```python
from build123d import *

# Parameters (mm, degrees)
FILLET1_R = 3


with BuildPart() as part:
    # Sketch1 → Revolve1 (revolve)
    with BuildSketch(Plane(origin=(0, 0, 0), x_dir=(0, 0, -1), z_dir=(1, 0, 0))):
        Polygon((-26, 0), (-15, 0), (-15, 2), (0, 2), (0, 12.5), (-4, 12.5), (-26, 9.408101637), align=None)
    revolve(axis=Axis((0, 0, 0), (0, 0, 1)))

    # Fillet1
    fillet1_edges = [part.edges().sort_by_distance(p)[0] for p in [
        (0, -9.408101637, 26),
        (0, -12.5, 4),
    ]]
    fillet(fillet1_edges, radius=FILLET1_R)


solid = part.part
```
Here's how the part is built. I have some questions about the finished solid (model axes, mm). Coordinates: 2 decimals unless noted, no trailing zeros. Order: outer loops, then holes, each group sorted by start corner. A loop starts at its lowest first (then second) coordinate and runs counter-clockwise, first axis right, second up.
1) Imagine slicing it at B-B on z = 23. List the corners of the cut face in (x, y) for me.
2) Imagine slicing it at A-A on z = 6.25. List the corners of the cut face in (x, y) for me, and give its area (3 significant figures).
3) Imagine slicing it at D-D on z = 16.75. List the corners of the cut face in (x, y) for me, and give its area (3 significant figures).
4) We'd pull the mould along X, two halves only. Please class faces 1 (the face through (3, 0, 0)), 2 (the face through (2, 0, 7)), 3 (the face through (-3.245, 10.303, 16.082)), 4 (the face through (0, 0, 15)): +X half, -X half, draft (parallel to the pull), parting line (faces both ways), or undercut.
5) Imagine slicing it at C-C on z = 9.5. List the corners of the cut face in (x, y) for me.
6) Will these pins go through, and if not, where does the flat tip stop? pin 1 (2 mm diameter, centred on x = -0.5, y = 0, fed in from -Z); pin 2 (1.5 mm diameter, centred on y = -0.5, z = 10, fed in from +X); pin 3 (1 mm diameter, centred on x = -3.5, z = 14.5, fed in from -Y).
7) I need wall thicknesses on line 1 (X direction, y = 0, z = 10.5); line 2 (Y direction, x = 0, z = 6); line 3 (Y direction, x = 1, z = 5). Which ranges of each line are inside material? Lowest first, please.
Response values:
1. outline: circle Ø19.66 at (0, 0)
2. outline: circle Ø24.37 at (0, 0); hole circle Ø4 at (0, 0)
2. area: 454 mm2
3. outline: circle Ø21.42 at (0, 0)
3. area: 360 mm2
4. face 1: draft
4. face 2: undercut
4. face 3: parting line
4. face 4: undercut
5. outline: circle Ø23.45 at (0, 0); hole circle Ø4 at (0, 0)
6. pin 1: stops at z = 15
6. pin 2: stops at x = 11.75
6. pin 3: stops at y = -10.63
7. line 1: x = -11.59 to -2, 2 to 11.59
7. line 2: y = -12.22 to -2, 2 to 12.22
7. line 3: y = -12.32 to -1.73, 1.73 to 12.32
